Here's how the part is built. I have some questions about the finished solid (model axes, mm). Coordinates: 2 decimals unless noted, no trailing zeros. Order: outer loops, then holes, each group sorted by start corner. A loop starts at its lowest first (then second) coordinate and runs counter-clockwise, first axis right, second up. Notation, with made-up numbers: (74.25, -11) - (94.25, -11) arc R38 cw to (94.25, 27) - close; hole circle Ø10 at (13, 80.5). An arc over 180 degrees is marked (long way). Answer in a Markdown table with one row per item. Add a question column.
Item 1: Will these pins go through, and if not, where does the flat tip stop? pin 1 Ø5 at (x, z) = (2.764, 37) entering from -Y; pin 2 Ø1.2 at (y, z) = (3, 24.5) entering from -X; pin 3 Ø1 at (y, z) = (3, 88) entering from -X; pin 4 Ø2 at (x, y) = (-28.5, 3) entering from +Z.
Item 2: I want a section at B-B (z = -93). Please give me the cut outline in (x, y).
Item 3: I want a section at C-C (y = 1.6). Count the separate pieces of the cut face and the enclosed holes in it, plus the area to 3 significant figures.
Item 4: I want a section at A-A (x = -10). Please give me the cut outline in (y, z).
Item 5: If I drill on line 1 along X through (y, z) = (1.5, 37); line 2 along X through (y, z) = (1.6, -57); line 3 along Z through (x, y) = (-0.5, 3.15), over which ranges is the centre line in solid material (lowest first)? Write a range as from..to.
Autodesk Inventor part; units mm, degrees
ref_plane "YZ Plane" through (0, 0, 0) normal (1, 0, 0) x (0, 1, 0)
ref_plane "XZ Plane" through (0, 0, 0) normal (0, 1, 0) x (-1, 0, 0)
ref_plane "XY Plane" through (0, 0, 0) normal (0, 0, 1) x (1, 0, 0)
sketch "Эскиз1" plane through (2.236, 0, -46.8876) normal (0, 1, 0) x (-1, 0, 0)
  line L0 (-10.528, 98.8876) -> (15, 98.8876)
  line L1 (15, 98.8876) -> (15, -5.1124)
  line L2 (15, -5.1124) -> (-10.528, -5.1124)
  line L3 (-10.528, -5.1124) -> (-10.528, 98.8876)
  point P0 (0, 0)
  dimension "d0" = 25.528
  dimension "d1" = 104
extrude "Выдавливание1" add sketch "Эскиз1" along normal blind 4
sketch "Эскиз2" plane through (2.236, 4, -46.8876) normal (0, 1, 0) x (0, 0, -1)
  circle A0 centre (-9.8876, -0.528) radius 2
  circle A1 centre (-83.8876, -0.528) radius 2
  point P0 (0, 0)
extrude "Выдавливание2" cut sketch "Эскиз2" against normal blind 4
sketch "Эскиз3" plane through (2.236, 4, -46.8876) normal (0, 1, 0) x (1, 0, 0)
  line L0 (-75, -191.6906) -> (-15, -191.6906)
  line L1 (-15, -191.6906) -> (-15, 97.9154)
  line L2 (-15, 97.9154) -> (-75, 97.9154)
  line L3 (-75, 97.9154) -> (-75, -191.6906)
  line L4 (-15, -98.8876) -> (10.528, -98.8876)
  line L5 (10.528, 5.1124) -> (-15, 5.1124)
  point P0 (-2.236, -46.8876)
  dimension "d8" = 92.803
  dimension "d9" = 92.803
  dimension "d10" = 60
extrude "Выдавливание3" add sketch "Эскиз3" against normal blind 4
sketch "Эскиз4" plane through (2.236, 4, -46.8876) normal (0, 1, 0) x (1, 0, 0)
  line L0 (-75, -191.6906) -> (-75, 97.9154)
  line L1 (-75, -191.6906) -> (-105, -109.2663)
  line L2 (-105, -109.2663) -> (-105, 97.9154)
  line L3 (-105, 97.9154) -> (-75, 97.9154)
  line L4 (-2.236, -46.8876) -> (-20.0662, -46.8876)
  dimension "d13" = 30
  dimension "d14" = 90
  dimension "d17" = 20
extrude "Выдавливание4" add sketch "Эскиз4" against normal blind 4
sketch "Эскиз5" plane through (-12.764, 0, 144.803) normal (0, 0, 1) x (1, 0, 0)
  line L0 (-60, 4) -> (0, 4)
  line L1 (0, 0) -> (-60, 0)
  line L2 (-60, 4) -> (-48, 4)
  line L3 (-48, 4) -> (-48, 0)
  line L4 (-48, 0) -> (-60, 0)
  line L5 (-60, 0) -> (-60, 4)
  point P0 (12.764, 0)
  dimension "d18" = 12
extrude "Выдавливание5" add sketch "Эскиз5" along normal blind 4
pattern_linear "Прямоуг.массив1" count 3 spacing 24 along (1, 0, 0) of "Выдавливание5"
sketch "Эскиз6" plane through (-12.764, 0, -144.803) normal (0, 0, -1) x (-1, 0, 0)
  line L0 (90, 4) -> (60, 4)
  line L1 (60, 0) -> (90, 0)
  line L2 (90, 4) -> (80, 4)
  line L3 (80, 4) -> (80, 0)
  line L4 (80, 0) -> (90, 0)
  line L5 (90, 0) -> (90, 4)
  point P0 (-12.764, 0)
  point P1 (90, 0)
  point P2 (80, 4)
  dimension "d24" = 10
extrude "Выдавливание6" add sketch "Эскиз6" along normal blind 4
pattern_linear "Прямоуг.массив2" count 5 spacing 20 along (1, 0, 0) of "Выдавливание6"
sketch "Эскиз7" plane through (2.236, 4, -46.8876) normal (0, 1, 0) x (1, 0, 0)
  line L0 (-105, 101.9154) -> (-105, -109.2663)
  line L1 (-105, 101.9154) -> (-109, 101.9154)
  line L2 (-109, 101.9154) -> (-109, 91.9154)
  line L3 (-109, 91.9154) -> (-105, 91.9154)
  line L4 (-105, 91.9154) -> (-105, 101.9154)
  point P0 (-2.236, -46.8876)
  dimension "d30" = 4
  dimension "d31" = 10
extrude "Выдавливание7" add sketch "Эскиз7" against normal blind 4
pattern_linear "Прямоуг.массив3" count 11 spacing 20 along (0, 0, 1) of "Выдавливание7"
sketch "Эскиз8" plane through (2.236, 0, -46.8876) normal (0, -1, 0) x (1, 0, 0)
  circle A0 centre (-36.9996, -88.3965) radius 2
  circle A1 centre (-36.9996, 182.1718) radius 2
  point P0 (-2.236, 46.8876)
extrude "Выдавливание8" cut sketch "Эскиз8" against normal blind 4
sketch "Эскиз9" plane through (-102.764, 0, 62.3787) normal (-0.9397, 0, 0.342) x (0.342, 0, 0.9397)
  line L0 (0, 4) -> (0, 0)
  line L1 (0, 4) -> (5, 4)
  line L2 (5, 4) -> (5, 0)
  line L3 (5, 0) -> (0, 0)
  line L4 (0, 0) -> (0, 4)
  point P0 (-23.4694, 0)
  dimension "d39" = 5
  dimension "d40" = 4
extrude "Выдавливание9" add sketch "Эскиз9" along normal blind 4
pattern_linear "Прямоуг.массив4" count 9 spacing 10 along (0.342, 0, 0.9397) of "Выдавливание9"
sketch "Эскиз10" plane through (2.236, 4, -46.8876) normal (0, 1, 0) x (1, 0, 0)
  line L0 (-109, 101.9154) -> (-109, 91.9154)
  line L1 (-109, 101.9154) -> (-105, 101.9154)
  line L2 (-105, 101.9154) -> (-105, -23.0846)
  line L3 (-105, -23.0846) -> (-109, -23.0846)
  line L4 (-109, -23.0846) -> (-109, 101.9154)
  point P0 (-2.236, -46.8876)
  dimension "d46" = 125
extrude "Выдавливание10" add sketch "Эскиз10" against normal blind 4
properties part number "KB33-046-004-008 - Центральная правая боковая пластина"
Values follow:
| question | item | result |
|---|---|---|
| 1 | pin 1 | stops at y = 0 |
| 1 | pin 2 | stops at x = -102.76 |
| 1 | pin 3 | stops at x = -93.62 |
| 1 | pin 4 | stops at z = 144.8 |
| 2 | outline | (-106.76, 0) - (-12.76, 0) - (-12.76, 4) - (-106.76, 4) - close |
| 3 | separate pieces | 1 |
| 3 | enclosed holes | 4 |
| 3 | area | 28,600 mm^2 |
| 4 | outline | (0, -52) - (4, -52) - (4, 52) - (0, 52) - close |
| 5 | line 1 | x = -106.76..0.76, 4.76..12.76 |
| 5 | line 2 | x = -106.76..-12.76 |
| 5 | line 3 | z = -52..52 |
